Source: CAD feature listing. Evaluate the final solid. Frame: model axes, mm. Round coordinates to 2 decimals unless told otherwise and drop trailing zeros. Loops run counter-clockwise (first coordinate to the right, second up) from the corner with the lowest first, then second, coordinate; pieces in that order, holes last. Notation, with made-up numbers: M -14,-8.75 L -4,-8.75 A33 ccw -4,30.25 Z; hole C -24,26 d11. An arc over 180 degrees is marked long. Answer as CSV lines item,"result". Start each with the question number.
```python
from build123d import *

# Parameters (mm, degrees)
CROQUIS1_R              = 60
SALIENTE_EXTRUIR1_DEPTH = 240
CROQUIS4_R              = 20
SALIENTE_EXTRUIR2_DEPTH = 335.410197
CROQUIS5_R              = 20
SALIENTE_EXTRUIR3_DEPTH = 335.410197
CROQUIS6_R              = 10
CORTAR_EXTRUIR2_DEPTH   = 335.410197
CROQUIS7_R              = 10
CORTAR_EXTRUIR3_DEPTH   = 335.410197
CROQUIS8_R              = 30
CORTAR_EXTRUIR4_DEPTH   = 304


with BuildPart() as part:
    # Croquis1 → Saliente-Extruir1 (new body)
    with BuildSketch(Plane.XY):
        Circle(CROQUIS1_R)
    extrude(amount=SALIENTE_EXTRUIR1_DEPTH)

    # Croquis4 → Saliente-Extruir2 (add)
    with BuildSketch(Plane(origin=(102, 0, -51), x_dir=(-0.44721359549995804, 0, -0.8944271909999159), z_dir=(0.8944271909999159, 0, -0.44721359549995804))):
        with Locations((-107.33126292, 0)):
            Circle(CROQUIS4_R)
    extrude(amount=-SALIENTE_EXTRUIR2_DEPTH)

    # Croquis5 → Saliente-Extruir3 (add)
    with BuildSketch(Plane(origin=(198, 0, 99), x_dir=(0.44721359549995826, 0, -0.8944271909999157), z_dir=(0.8944271909999157, 0, 0.44721359549995826))):
        with Locations((-107.33126292, 0)):
            Circle(CROQUIS5_R)
    extrude(amount=-SALIENTE_EXTRUIR3_DEPTH)

    # Croquis6 → Cortar-Extruir2 (cut)
    with BuildSketch(Plane(origin=(198, 0, 99), x_dir=(0.44721359549995826, 0, -0.8944271909999157), z_dir=(0.8944271909999157, 0, 0.44721359549995826))):
        with Locations((-107.33126292, 0)):
            Circle(CROQUIS6_R)
    extrude(amount=-CORTAR_EXTRUIR2_DEPTH, mode=Mode.SUBTRACT)

    # Croquis7 → Cortar-Extruir3 (cut)
    with BuildSketch(Plane(origin=(102, 0, -51), x_dir=(-0.44721359549995804, 0, -0.8944271909999159), z_dir=(0.8944271909999159, 0, -0.44721359549995804))):
        with Locations((-107.33126292, 0)):
            Circle(CROQUIS7_R)
    extrude(amount=-CORTAR_EXTRUIR3_DEPTH, mode=Mode.SUBTRACT)

    # Croquis8 → Cortar-Extruir4 (cut)
    with BuildSketch(Plane(origin=(0, 0, 0), x_dir=(-1, 0, 0), z_dir=(0, 0, -1))):
        Circle(CROQUIS8_R)
    extrude(amount=-CORTAR_EXTRUIR4_DEPTH, mode=Mode.SUBTRACT)


solid = part.part
```
1) Section B-B, the plane z = 31. Give the number of separate pieces and of enclosed holes in the cut face, and give its area (3 significant figures).
2) Section A-A, the plane x = 0. Return loops of the section in (y, z), and give its area (3 significant figures).
3) Ray query, line 1 along Y through (x, z) = (0, 65.5); line 2 along X through (y, z) = (18.5, 123); line 3 along Z through (x, y) = (32, -5.5). Return the intervals inside material, ascending.
4) Contact query for flat-ended pins moving along their axis: pin 1 Ø3 at (y, z) = (-37, 158) entering from +X; pin 2 Ø8 at (x, z) = (-104.5, 175) entering from -Y; pin 3 Ø8 at (x, z) = (-34.5, 73.5) entering from +Y. Output: stop coordinate, or through.
5) Mould query, pull axis Z, two halves, no side actions, for faces 1 (the cylindrical face through (-91.36, 0.44, 85.49)), 2 (the flat face through (12, 28, 240)), 3 (the flat face through (154, 5, 53)). Classes: pulls with the +Z half, pulls with the -Z half, needs draft (parallel to the pull), parting line crosses it, or undercut.
Findings below:
1,separate pieces,"3"
1,enclosed holes,"1"
1,area,"8,810 mm²"
2,outline,"M -60,0 L -30,0 L -30,240 L -60,240 Z; M 30,0 L 60,0 L 60,240 L 30,240 Z"
2,area,"14,400 mm²"
3,line 1,"-60 to -30, 30 to 60"
3,line 2,"-57.08 to -23.62, 23.62 to 57.08"
3,line 3,"0 to 94.66, 113.34 to 126.66, 145.34 to 240"
4,pin 1,"x = 48.37"
4,pin 2,"y = -20"
4,pin 3,"y = 51.67"
5,face 1,"undercut"
5,face 2,"pulls with the +Z half"
5,face 3,"pulls with the -Z half"
